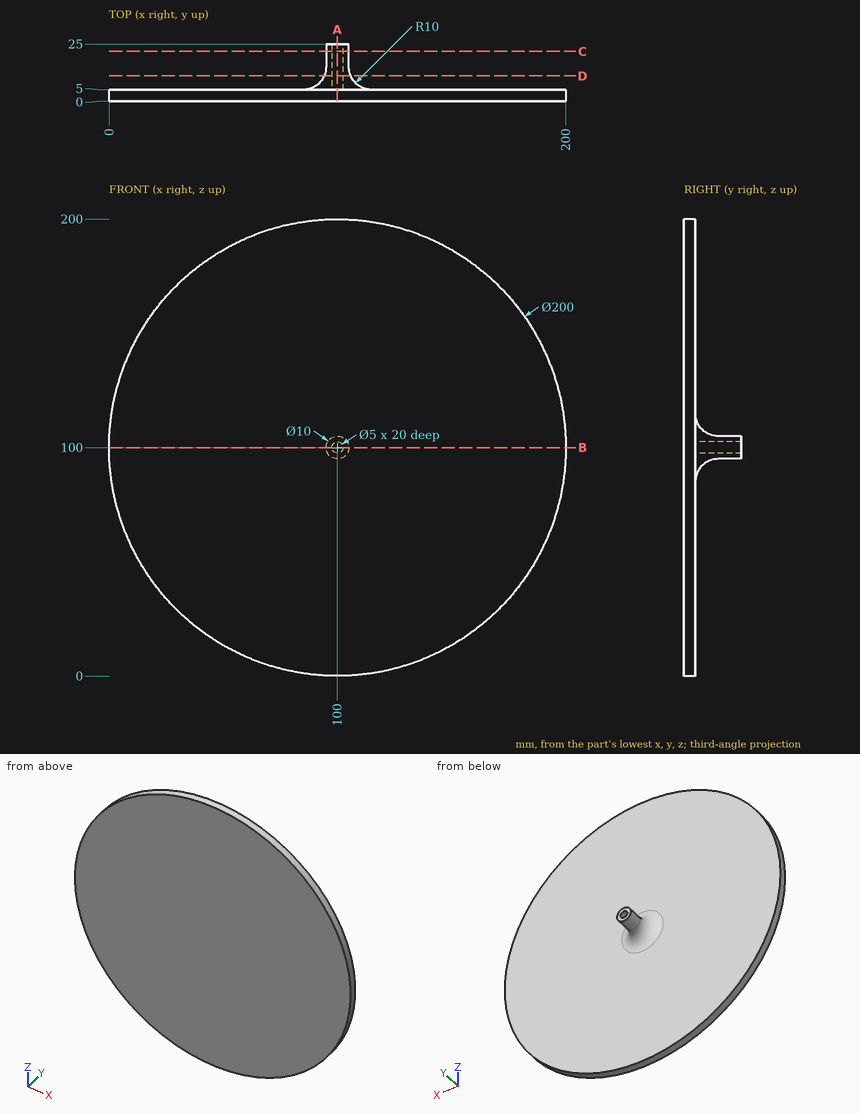
Answer from the drawing. Dimensions are ordinates in mm from the lowest x, y and z of the part. Give positions to 0.01 mm unless a question says otherwise; leave off trailing zeros. Write each loop counter-clockwise with the first axis right and the second up, starting at its lowest first coordinate (ties: lowest second). Pieces come first, ordered by that corner, then holes. Notation, with made-up numbers: (63, -10.75) - (71, -10.75) arc R20 cw to (71, 14.25) - close; hole circle Ø8 at (43, 64.5). An arc over 180 degrees is marked (long way). Answer in a Markdown table with one row per item. Add a question column.
Item 1: Find the intervals of material crossed by L1, parallel to Z at x = 100, y = 20.75; L2, parallel to Y at x = 51.5, z = 85, in increasing order.
Item 2: Flat-ended cylindrical pins translate along their axes: P1, Ø6, axis at x = 157.5, y = 4.5, coming from the -Z side; P2, Ø1.5, axis at x = 64.5, z = 85, coming from the +Y side; P3, Ø8, axis at x = 88, y = 13, coming from the -Z side; P4, Ø10, axis at y = 8.5, z = 152.5, coming from the -X side. Find the tip coordinate at first contact, or state that the pin passes through.
Item 3: Section A-A, the plane x = 100 is taken. Write down the section's boundary in (y, z).
Item 4: Section D-D, the plane y = 11 is taken. Write down the section's boundary in (x, z).
Item 5: Section C-C, the plane y = 21.75 is taken. Write down the section's boundary in (x, z).
Item 6: Section B-B, the plane z = 100 is taken. Write down the section's boundary in (x, y), and give its area (3 significant figures).
Recorded:
| question | item | result |
|---|---|---|
| 1 | L1 | z = 95 to 97.5, 102.5 to 105 |
| 1 | L2 | y = 0 to 5 |
| 2 | P1 | stops at z = 16.16 |
| 2 | P2 | stops at y = 5 |
| 2 | P3 | passes through |
| 2 | P4 | stops at x = 12.79 |
| 3 | outline | (0, 0) - (5, 0) - (5, 85) arc R10 cw to (15, 95) - (25, 95) - (25, 97.5) - (5, 97.5) - (5, 102.5) - (25, 102.5) - (25, 105) - (15, 105) arc R10 cw to (5, 115) - (5, 200) - (0, 200) - close |
| 4 | outline | circle Ø11.67 at (100, 100); hole circle Ø5 at (100, 100) |
| 5 | outline | circle Ø10 at (100, 100); hole circle Ø5 at (100, 100) |
| 6 | outline | (0, 0) - (200, 0) - (200, 5) - (115, 5) arc R10 cw to (105, 15) - (105, 25) - (102.5, 25) - (102.5, 5) - (97.5, 5) - (97.5, 25) - (95, 25) - (95, 15) arc R10 cw to (85, 5) - (0, 5) - close |
| 6 | area | 1,140 mm2 |
